from build123d import *

# Parameters (mm, degrees)
EXTRUDE_1_DEPTH     = 52
EXTRUDE_2_DEPTH     = 2.5
EXTRUDE_3_DEPTH     = 2.5
SKETCH_4_R          = 1.6
SKETCH_4_R_2        = 12.5
CUT_EXTRUDE_1_DEPTH = 5
SKETCH_6_R          = 1.6
CUT_EXTRUDE_2_DEPTH = 5
CUT_EXTRUDE_3_DEPTH = 136.636948309


with BuildPart() as part:
    # 草图1 → 凸台-拉伸1 (new body)
    with BuildSketch(Plane.XY):
        Polygon((32.526911935, 70.711610456), (0, 38.184698521), (0, 0), (100.73852239, 0), (100.73852239, 2.5), (94.853312534, 2.5), (2.5, 2.5), (2.5, 37.149164615), (32.494813779, 67.143978395), (34.294678888, 68.943843503), align=None)
    extrude(amount=EXTRUDE_1_DEPTH)

    # 草图2 → 凸台-拉伸2 (add)
    with BuildSketch(Plane.XY.offset(52)):
        Polygon((32.526911935, 70.711610456), (0, 38.184698521), (0, 0), (100.73852239, 0), (100.73852239, 1), (34.294678888, 68.943843503), align=None)
    extrude(amount=EXTRUDE_2_DEPTH)

    # 草图3 → 凸台-拉伸3 (add)
    with BuildSketch(Plane(origin=(0, 0, 0), x_dir=(-1, 0, 0), z_dir=(0, 0, -1))):
        Polygon((-32.526911935, 70.711610456), (0, 38.184698521), (0, 0), (-100.73852239, 0), (-100.73852239, 2.5), (-34.294678888, 68.943843503), align=None)
    extrude(amount=EXTRUDE_3_DEPTH)

    # 草图4 → 切除-拉伸1 (cut)
    with BuildSketch(Plane(origin=(-19.092349261, 19.092349261, 0), x_dir=(0, 0, 1), z_dir=(-0.7071067811865468, 0.7071067811865483, 0))):
        with Locations(Location((10.5, 67.500659262, 0), (0, 0, 270))):
            Circle(SKETCH_4_R)
        with Locations(Location((41.5, 67.500659262, 0), (0, 0, 270))):
            Circle(SKETCH_4_R)
        with Locations(Location((10.5, 36.500659262, 0), (0, 0, 270))):
            Circle(SKETCH_4_R)
        with Locations(Location((41.5, 36.500659262, 0), (0, 0, 270))):
            Circle(SKETCH_4_R)
        with Locations(Location((26, 52.000659262, 0), (0, 0, 270))):
            Circle(SKETCH_4_R_2)
    extrude(amount=-CUT_EXTRUDE_1_DEPTH, mode=Mode.SUBTRACT)

    # 草图6 → 切除-拉伸2 (cut)
    with BuildSketch(Plane.XZ):
        with Locations(Location((10, 48.5, 0), (0, 0, 270))):
            Circle(SKETCH_6_R)
        with Locations(Location((10, 3.5, 0), (0, 0, 270))):
            Circle(SKETCH_6_R)
        with Locations(Location((39.092556486, 41.177216573, 0), (0, 0, 270))):
            Circle(SKETCH_6_R)
        with Locations(Location((39.092556486, 10.822783427, 0), (0, 0, 270))):
            Circle(SKETCH_6_R)
    extrude(amount=-CUT_EXTRUDE_2_DEPTH, mode=Mode.SUBTRACT)

    # 草图7 → 切除-拉伸3 (cut, through all)
    with BuildSketch(Plane.XY.offset(54.5)):
        Polygon((61, 42.23852239), (61, 0), (103.406412913, 0), (103.406412913, 12.738477269), align=None)
    extrude(amount=-CUT_EXTRUDE_3_DEPTH, mode=Mode.SUBTRACT)


solid = part.part
The listing builds one solid part. Answer for the finished solid, in the listing's coordinates (mm). A direction names the side the tool comes from. Give positions to 0.01 mm unless a question says otherwise; leave off trailing zeros. Write each loop counter-clockwise with the first axis right and the second up, starting at its lowest first coordinate (ties: lowest second). Pieces come first, ordered by that corner, then holes.
Item 1: Section A-A, the plane z = 48.5 is taken. Write down the section's boundary in (x, y).
Item 2: Section C-C, the plane x = 45.5 is taken. Write down the section's boundary in (y, z).
Item 3: Find the intervals of material crossed by line 1 along Z through (x, y) = (22.5, 3); line 2 along Y through (x, z) = (19, 3.5); line 3 along Z through (x, y) = (51, 52), in increasing order.
Item 4: Section D-D, the plane z = 27 is taken. Write down the section's boundary in (x, y), plus the area to 3 significant figures.
Item 5: Which of the six approach directions +Z, -Z, +X, -X, +Y, -Y give full straight-line access (tool end or side, diameter ignored) to faces 1 (the cylindrical face through (10.38, 46.83, 21.21)), 2 (the flat face through (47.834, 55.099, 53.232)), 3 (the flat face through (30, 0, 26)), 4 (the flat face through (32, 2.5, 26)), 5 (the cylindrical face through (8.58, 1.23, 2.76))?
Item 6: Flat-ended cylindrical pins translate along their axes: P1, Ø5, axis at y = 44.5, z = 34, coming from the -X side; P2, Ø12, axis at y = 13, z = 40, coming from the +X side; P3, Ø1.9, axis at x = 10, z = 48.5, coming from the +Y side. Find the tip coordinate at first contact, or state that the pin passes through.
Item 7: Section B-B, the plane y = 9 is taken. Write down the section's boundary in (x, z).
Item 8: Determine the mould class of faces 6 (the flat face through (9.263, 47.448, 32.732)), 7 (the flat face through (31, 29, 52)), 8 (the flat face through (30, 28, -2.5)) for opening direction Y: released by +Y, released by -Y, zero draft, split by the parting line, or undercut.
Completed:
1. outline: (0, 0) - (8.4, 0) - (8.4, 2.5) - (2.5, 2.5) - (2.5, 37.15) - (34.29, 68.94) - (32.53, 70.71) - (0, 38.18) - close; (11.6, 0) - (61, 0) - (61, 2.5) - (11.6, 2.5) - close
2. outline: (0, -2.5) - (57.74, -2.5) - (57.74, 0) - (2.5, 0) - (2.5, 52) - (57.49, 52) - (57.49, 54.5) - (0, 54.5) - close
3. line 1: z = -2.5 to 0, 52 to 54.5
3. line 2: y = 0 to 2.5, 53.65 to 57.18
3. line 3: z = -2.5 to 0
4. outline: (0, 0) - (61, 0) - (61, 2.5) - (2.5, 2.5) - (2.5, 37.15) - (10.63, 45.28) - (8.87, 47.05) - (0, 38.18) - close; (26.49, 64.67) - (28.26, 62.91) - (34.29, 68.94) - (32.53, 70.71) - close
4. area: 292 mm2
5. face 1: none
5. face 2: +Z, +X, +Y
5. face 3: +Z, -Z, +X, -X, -Y
5. face 4: +X
5. face 5: -Y
6. P1: stops at x = 3.82
6. P2: stops at x = 2.5
6. P3: stops at y = 49.13
7. outline: (0, -2.5) - (61, -2.5) - (61, 0) - (2.5, 0) - (2.5, 52) - (61, 52) - (61, 54.5) - (0, 54.5) - close
8. face 6: released by +Y
8. face 7: undercut
8. face 8: zero draft
